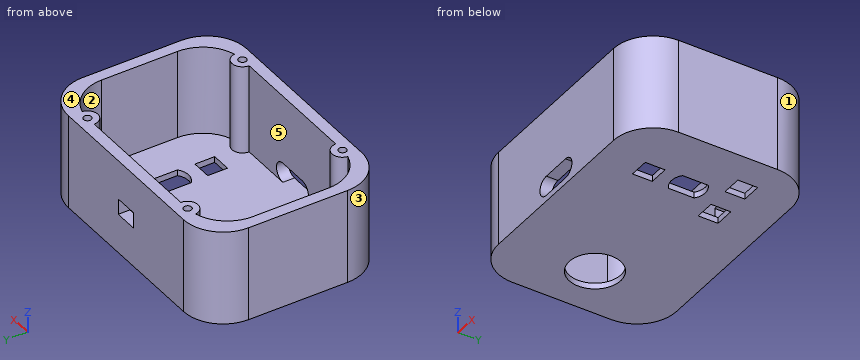
from build123d import *

# Parameters (mm, degrees)
SKETCH1_W           = 130
SKETCH1_H           = 90
BOSS_EXTRUDE1_DEPTH = 48
FILLET1_R           = 20
CUT_EXTRUDE4_DEPTH  = 45
SKETCH3_R           = 5.240734637
SKETCH3_R_2         = 5.258413594
BOSS_EXTRUDE2_DEPTH = 45
CUT_EXTRUDE5_REACH  = 92
SKETCH4_W           = 12
SKETCH4_H           = 8
SKETCH5_R           = 2
CUT_EXTRUDE6_DEPTH  = 23
CUT_EXTRUDE7_DEPTH  = 10
SKETCH7_R           = 13
CUT_EXTRUDE8_DEPTH  = 10
SKETCH8_W           = 10
SKETCH8_H           = 10
CUT_EXTRUDE9_DEPTH  = 30
SKETCH9_W           = 10
SKETCH9_H           = 10
CUT_EXTRUDE10_DEPTH = 10
CUT_EXTRUDE11_DEPTH = 10


with BuildPart() as part:
    # Sketch1 → Boss-Extrude1 (new body)
    with BuildSketch(Plane.XY):
        with Locations((65, 45)):
            Rectangle(SKETCH1_W, SKETCH1_H)
    extrude(amount=BOSS_EXTRUDE1_DEPTH)

    # Fillet1
    fillet1_edges = [part.edges().sort_by_distance(p)[0] for p in [
        (0, 90, 24),
        (130, 90, 24),
        (130, 0, 24),
        (0, 0, 24),
    ]]
    fillet(fillet1_edges, radius=FILLET1_R)

    # Sketch2 → Cut-Extrude4 (cut)
    with BuildSketch(Plane.XY.offset(48)):
        with BuildLine():
            Line((104.142135624, 5.857864376), (25.857864376, 5.857864376))
            ThreePointArc((25.857864376, 5.857864376), (11.715728753, 11.715728753), (5.857864376, 25.857864376))
            Line((5.857864376, 25.857864376), (5.857864376, 64.142135624))
            ThreePointArc((5.857864376, 64.142135624), (11.715728753, 78.284271247), (25.857864376, 84.142135624))
            Line((25.857864376, 84.142135624), (104.142135624, 84.142135624))
            ThreePointArc((104.142135624, 84.142135624), (118.284271247, 78.284271247), (124.142135624, 64.142135624))
            Line((124.142135624, 64.142135624), (124.142135624, 25.857864376))
            ThreePointArc((124.142135624, 25.857864376), (118.284271247, 11.715728753), (104.142135624, 5.857864376))
        make_face()
    extrude(amount=-CUT_EXTRUDE4_DEPTH, mode=Mode.SUBTRACT)

    # Sketch3 → Boss-Extrude2 (add)
    with BuildSketch(Plane.XY.offset(3)):
        with Locations((25.857864376, 84.142135624)):
            Circle(SKETCH3_R)
        with Locations((104.142135624, 84.142135624)):
            Circle(SKETCH3_R)
        with Locations((25.857864376, 5.857864376)):
            Circle(SKETCH3_R_2)
        with Locations((104.142135624, 5.857864376)):
            Circle(SKETCH3_R)
    extrude(amount=BOSS_EXTRUDE2_DEPTH)

    # Sketch4 → Cut-Extrude5 (cut, up to next)
    with BuildSketch(Plane(origin=(0, 90, 0), x_dir=(1, 0, 0), z_dir=(0, 1, 0)), mode=Mode.PRIVATE) as cut_extrude5_sk1:
        with Locations((65, -24)):
            Rectangle(SKETCH4_W, SKETCH4_H)
    cut_extrude5_tool1 = extrude(cut_extrude5_sk1.sketch, amount=-CUT_EXTRUDE5_REACH, mode=Mode.PRIVATE) & part.part
    add(cut_extrude5_tool1.solids().sort_by_distance((65, 90, 24))[0], mode=Mode.SUBTRACT)

    # Sketch5 → Cut-Extrude6 (cut)
    with BuildSketch(Plane.XY.offset(48)):
        with Locations((25.857864376, 84.142135624)):
            Circle(SKETCH5_R)
        with Locations((104.142135624, 84.142135624)):
            Circle(SKETCH5_R)
        with Locations((104.142135624, 5.857864376)):
            Circle(SKETCH5_R)
        with Locations((25.857864376, 5.857864376)):
            Circle(SKETCH5_R)
    extrude(amount=-CUT_EXTRUDE6_DEPTH, mode=Mode.SUBTRACT)

    # Sketch6 → Cut-Extrude7 (cut)
    with BuildSketch(Plane.XY.offset(3)):
        with BuildLine():
            Line((93.401400986, 51.480740698), (93.401400986, 38.519259302))
            ThreePointArc((93.401400986, 38.519259302), (98.901400986, 36.5), (104.401400986, 38.519259302))
            Line((104.401400986, 38.519259302), (104.401400986, 51.480740698))
            ThreePointArc((104.401400986, 51.480740698), (98.901400986, 53.5), (93.401400986, 51.480740698))
        make_face()
    extrude(amount=-CUT_EXTRUDE7_DEPTH, mode=Mode.SUBTRACT)

    # Sketch7 → Cut-Extrude8 (cut)
    with BuildSketch(Plane.XY.offset(3)):
        with Locations((25.857864376, 45)):
            Circle(SKETCH7_R)
    extrude(amount=-CUT_EXTRUDE8_DEPTH, mode=Mode.SUBTRACT)

    # Sketch8 → Cut-Extrude9 (cut)
    with BuildSketch(Plane(origin=(0, 0, 0), x_dir=(-1, 0, 0), z_dir=(0, 0, -1))):
        with Locations((-109.401400986, 65)):
            Rectangle(SKETCH8_W, SKETCH8_H)
        with Locations((-88.401400986, 65)):
            Rectangle(SKETCH8_W, SKETCH8_H)
    extrude(amount=-CUT_EXTRUDE9_DEPTH, mode=Mode.SUBTRACT)

    # Sketch9 → Cut-Extrude10 (cut)
    with BuildSketch(Plane(origin=(0, 0, 0), x_dir=(-1, 0, 0), z_dir=(0, 0, -1))):
        with Locations((-98.901400986, 25)):
            Rectangle(SKETCH9_W, SKETCH9_H)
    extrude(amount=-CUT_EXTRUDE10_DEPTH, mode=Mode.SUBTRACT)

    # Sketch11 → Cut-Extrude11 (cut)
    with BuildSketch(Plane(origin=(0, 5.857864376, 0), x_dir=(1, 0, 0), z_dir=(0, 1, 0))):
        with BuildLine():
            Line((57.508839478, -3), (72.508839478, -3))
            ThreePointArc((72.508839478, -3), (77.508839478, -8), (72.508839478, -13))
            Line((72.508839478, -13), (57.508839478, -13))
            ThreePointArc((57.508839478, -13), (52.508839478, -8), (57.508839478, -3))
        make_face()
    extrude(amount=-CUT_EXTRUDE11_DEPTH, mode=Mode.SUBTRACT)


solid = part.part
Input: part model. Units: mm. Frame: model coordinates. Face numbers are marked on the shaded views. A direction names the side the tool comes from. Give positions to 0.01 mm unless a question says otherwise; leave off trailing zeros. Write each loop counter-clockwise with the first axis right and the second up, starting at its lowest first coordinate (ties: lowest second). Pieces come first, ordered by that corner, then holes. Notation, with made-up numbers: M 48.25,-1.5 L 75.25,-1.5 A23 ccw 75.25,36.5 Z; hole C 56,-18.75 d3. An arc over 180 degrees is marked long. Use one line per item in the form item = value.
1. First-contact query: P1, Ø1.8, axis at y = 86, z = 24, coming from the +X side; P2, Ø4, axis at y = 77.5, z = 30.5, coming from the -X side; P3, Ø10, axis at x = 56, y = 47.5, coming from the -Z side; P4, Ø2, axis at x = 104, y = 5.5, coming from the +Z side. Flat tips, straight axial feed; report the tip coordinate or a pass-through.
Outcome:
P1 = 123.11
P2 = 0.77
P3 = 0
P4 = 25
2. Cut plane D-D on x = 74.5. Return loops of the section in (y, z), and give its area (3 significant figures).
Outcome:
outline = M 0,0 L 90,0 L 90,48 L 84.14,48 L 84.14,3 L 5.86,3 L 5.86,3.41 L 0,3.41 Z; M 0,12.59 L 5.86,12.59 L 5.86,48 L 0,48 Z
area = 743 mm²
3. Mould query, pull axis Y, two halves, no side actions, for the marked faces 1, 2 and 3. Classes: released by +Y, released by -Y, zero draft, split by the parting line, or undercut.
Outcome:
face_1 = released by +Y
face_2 = undercut
face_3 = released by -Y
4. Reachability of the marked faces 4 and 5 from +Z, -Z, +X, -X, +Y, -Y: full face, straight path, thin tool, end or side. Return the list, or none.
Outcome:
face_4 = +Z, +X, -X, +Y, -Y
face_5 = +Z
5. Ray query, L1, parallel to X at y = 60.5, z = 2; L2, parallel to Y at x = 83, z = 23.5; L3, parallel to X at y = 26.5, z = 44.5. Return the intervals inside material, ascending.
Outcome:
L1 = 0 to 83.4, 93.4 to 104.4, 114.4 to 130
L2 = 0 to 5.86, 84.14 to 90
L3 = 0 to 5.86, 124.14 to 130
6. Cut plane A-A on y = 45. Return loops of the section in (x, z).
Outcome:
outline = M 0,0 L 12.86,0 L 12.86,3 L 5.86,3 L 5.86,48 L 0,48 Z; M 38.86,0 L 93.4,0 L 93.4,3 L 38.86,3 Z; M 104.4,0 L 130,0 L 130,48 L 124.14,48 L 124.14,3 L 104.4,3 Z
7. Cut plane B-B on z = 29.5. Return loops of the section in (x, y).
Outcome:
outline = M 0,20 A20 ccw 20,0 L 110,0 A20 ccw 130,20 L 130,70 A20 ccw 110,90 L 20,90 A20 ccw 0,70 Z; hole M 5.86,25.86 A20 ccw 20.65,6.55 A5.26 cw 31.12,5.86 L 98.9,5.86 A5.24 cw 109.34,6.54 A20 ccw 124.14,25.86 L 124.14,64.14 A20 ccw 109.34,83.46 A5.24 cw 98.9,84.14 L 31.1,84.14 A5.24 cw 20.66,83.46 A20 ccw 5.86,64.14 Z; hole C 25.86,5.86 d4; hole C 25.86,84.14 d4; hole C 104.14,5.86 d4; hole C 104.14,84.14 d4
8. Cut plane C-C on z = 8. Return loops of the section in (x, y), and give its area (3 significant figures).
Outcome:
outline = M 0,20 A20 ccw 20,0 L 52.51,0 L 52.51,5.86 L 31.12,5.86 A5.26 ccw 20.65,6.55 A20 cw 5.86,25.86 L 5.86,64.14 A20 cw 20.66,83.46 A5.24 ccw 31.1,84.14 L 98.9,84.14 A5.24 ccw 109.34,83.46 A20 cw 124.14,64.14 L 124.14,25.86 A20 cw 109.34,6.54 A5.24 ccw 98.9,5.86 L 77.51,5.86 L 77.51,0 L 110,0 A20 ccw 130,20 L 130,70 A20 ccw 110,90 L 20,90 A20 ccw 0,70 Z
area = 2,460 mm²
